Geometry check sheet. Reference: drawing and pictorial views, mm from the part's lowest x, y, z. A direction names the side the tool comes from. Round coordinates to 2 decimals unless told otherwise and drop trailing zeros. Write each loop counter-clockwise with the first axis right and the second up, starting at its lowest first coordinate (ties: lowest second). Pieces come first, ordered by that corner, then holes. Notation, with made-up numbers: M 12.5,20.5 L 53.5,20.5 A27 ccw 53.5,39.5 Z; hole C 81,37.5 d11. An arc over 180 degrees is marked long. One line per item, written item: value. Start each with the question number.
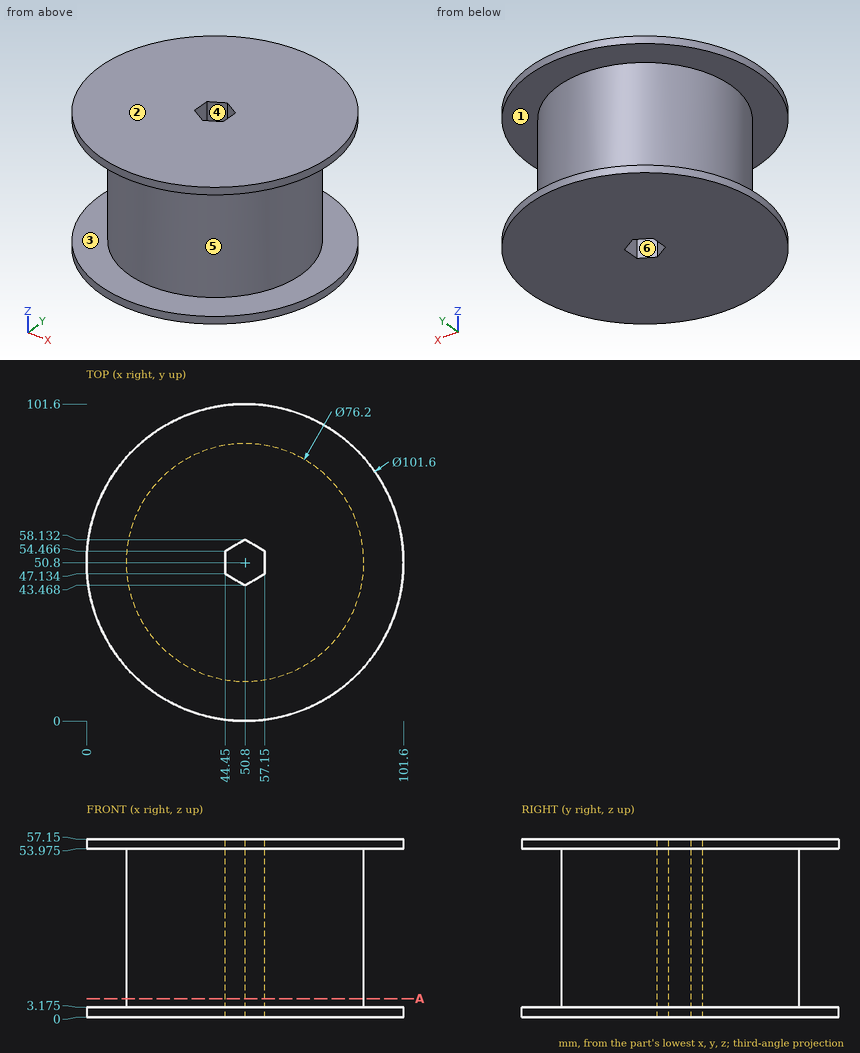
1) Cross-section at A-A (z = 6). Record the boundary of the cut face in (x, y).
2) Mould release check, pull along X, two halves, no side actions. Record for the marked faces 3, 4, 5 and 6: pulls with the +X half, pulls with the -X half, needs draft (parallel to the pull), parting line crosses it, or undercut.
3) Access from +Z, -Z, +X, -X, +Y, -Y to the whole of each face (thin tool, end or side, straight path). Record for the marked faces 1 and 2.
4) Gauge pin test, flat ends, axial feed: pin 1 Ø8 at (y, z) = (49.5, 27.5) entering from -X; pin 2 Ø6 at (y, z) = (28.5, 47) entering from -X; pin 3 Ø8 at (y, z) = (85, 15.5) entering from -X; pin 4 Ø1 at (x, y) = (17, 41) entering from -Z. Record the tip position at first contact, or that the pin passes through.
5) Thickness scan on line 1 (Y direction, x = 46.5, z = 52.5); line 2 (Y direction, x = 32, z = 37); line 3 (X direction, y = 22, z = 4.5) (1 decimal). Record the ranges inside material, lowest first.
Results below:
1. outline: C 50.8,50.8 d76.2; hole M 44.45,47.13 L 50.8,43.47 L 57.15,47.13 L 57.15,54.47 L 50.8,58.13 L 44.45,54.47 Z
2. face 3: needs draft
2. face 4: undercut
2. face 5: parting line crosses it
2. face 6: undercut
3. face 1: none
3. face 2: +Z, +X, -X, +Y, -Y
4. pin 1: stops at x = 12.7
4. pin 2: stops at x = 17.95
4. pin 3: stops at x = 27.57
4. pin 4: stops at z = 0
5. line 1: y = 12.94 to 45.95, 55.65 to 88.66
5. line 2: y = 17.66 to 83.94
5. line 3: x = 25.9 to 75.7
